Drawing for the job (mm, zero at the part's lowest x, y, z). A direction names the side the tool comes from. Give positions to 0.01 mm unless a question says otherwise; leave off trailing zeros. Loops run counter-clockwise (first coordinate to the right, second up) from the corner with the lowest first, then second, coordinate; pieces in that order, holes last. Notation, with made-up numbers: (51, 50) -> (104, 50) arc R19 cw to (104, 75) -> close; hole circle Ø2 at (-33.5, 52). An arc over 180 degrees is marked (long way). Use CSV: the item, a comma, the result in double quotes. Start each with the question number.
(1) 3-axis set-ups, long thin cutter, end or side, ignore diameter. For the marked faces 1 and 2: which of +Z, -Z, +X, -X, +Y, -Y reach the whole face in a straight line?
(2) Pull direction Y, two halves, no side cores. Call the marked faces 3, 4 and 5: pulls with the +Y half, pulls with the -Y half, needs draft (parallel to the pull), parting line crosses it, or undercut.
(3) Cut at A-A on y = 65. Write the cut outline in (x, z).
(4) Cut at B-B on x = 20. Write the cut outline in (y, z).
(5) Cut at C-C on z = 18. Write the cut outline in (x, y), then the cut area to 3 significant figures.
(6) Cut at D-D on x = 65. Write the cut outline in (y, z), then the cut area to 3 significant figures.
(7) Flat gauge pins, fed straight in: pin 1 (6 mm diameter, centred on x = 93.5, z = 6, fed in from +Y); pin 2 (3 mm diameter, centred on x = 54, z = 26, fed in from -Y) (1 decimal); pin 3 (1 mm diameter, centred on x = 41.5, y = 31.5, fed in from -Z); pin 4 (2 mm diameter, centred on x = 62, z = 45.5, fed in from +Y). Where does each tip first touch, or does it go through?
(8) Drill centre lines: probe 1 along Z at (x, y) = (75, 103.5); probe 2 along Y at (x, z) = (20, 10.75) (1 decimal); probe 3 along Y at (x, z) = (87.5, 3). Where is each one in solid material? Low to high.
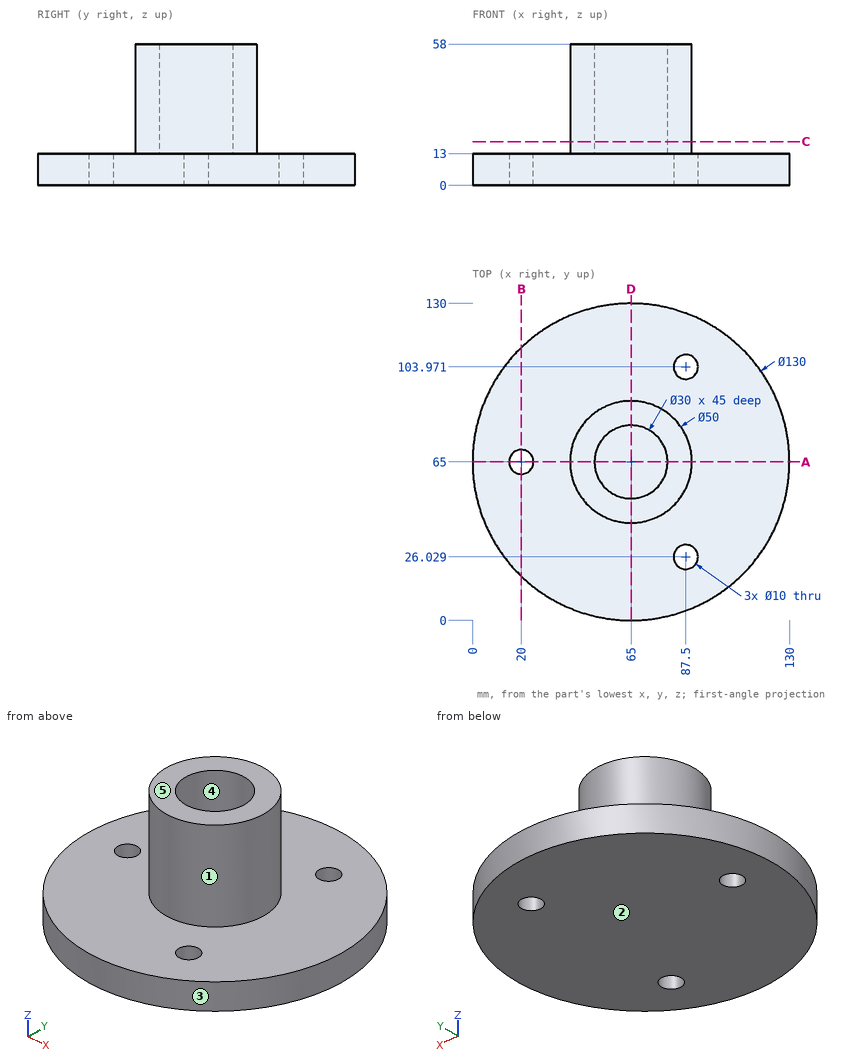
Check result:
1,face 1,"+Z"
1,face 2,"-Z, +X, -X, +Y, -Y"
2,face 3,"parting line crosses it"
2,face 4,"undercut"
2,face 5,"needs draft"
3,outline,"(0, 0) -> (15, 0) -> (15, 13) -> (0, 13) -> close; (25, 0) -> (130, 0) -> (130, 13) -> (90, 13) -> (90, 58) -> (80, 58) -> (80, 13) -> (50, 13) -> (50, 58) -> (40, 58) -> (40, 13) -> (25, 13) -> close"
4,outline,"(18.1, 0) -> (60, 0) -> (60, 13) -> (18.1, 13) -> close; (70, 0) -> (111.9, 0) -> (111.9, 13) -> (70, 13) -> close"
5,outline,"circle Ø50 at (65, 65); hole circle Ø30 at (65, 65)"
5,area,"1,260 mm²"
6,outline,"(0, 0) -> (130, 0) -> (130, 13) -> (90, 13) -> (90, 58) -> (80, 58) -> (80, 13) -> (50, 13) -> (50, 58) -> (40, 58) -> (40, 13) -> (0, 13) -> close"
6,area,"2,590 mm²"
7,pin 1,"y = 124.79"
7,pin 2,"y = 41.9"
7,pin 3,"z = 0"
7,pin 4,"y = 89.92"
8,probe 1,"0 to 13"
8,probe 2,"18.1 to 60, 70 to 111.9"
8,probe 3,"4.02 to 21.03, 31.03 to 98.97, 108.97 to 125.98"
